Work out the finished part from the listing and answer in its coordinate system (mm). Round coordinates to 2 decimals unless told otherwise and drop trailing zeros. Write each loop counter-clockwise with the first axis right and the second up, starting at its lowest first coordinate (ties: lowest second). Pieces come first, ordered by that corner, then holes. Notation, with made-up numbers: (-35, 74) -> (-3, 74) arc R23 cw to (-3, 108) -> close; hole circle Ø4 at (-39.5, 59). An arc over 180 degrees is marked (long way). Answer as a JSON object with one key per item and string values. Group by question number.
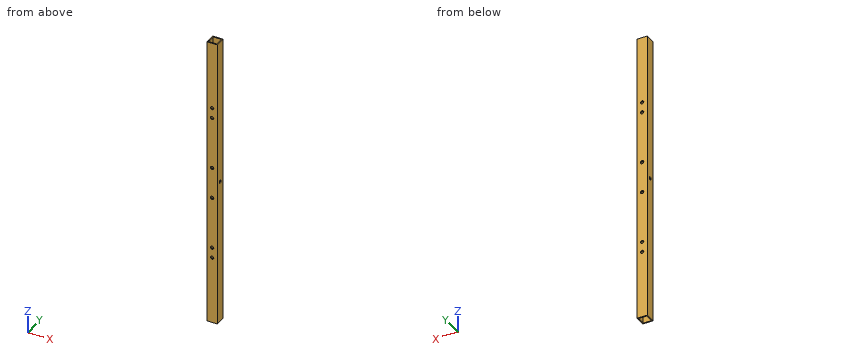
from build123d import *

# Parameters (mm, degrees)
SKETCH1_W           = 10
SKETCH1_H           = 10
SKETCH1_W_2         = 8
SKETCH1_H_2         = 8
BOSS_EXTRUDE1_DEPTH = 280
CUT_EXTRUDE1_REACH  = 282.223
SKETCH2_R           = 1.6
CUT_EXTRUDE2_REACH  = 282.223
SKETCH3_R           = 1.6


with BuildPart() as part:
    # Sketch1 → Boss-Extrude1 (new body)
    with BuildSketch(Plane.XY):
        Rectangle(SKETCH1_W, SKETCH1_H)
        Rectangle(SKETCH1_W_2, SKETCH1_H_2, mode=Mode.SUBTRACT)
    extrude(amount=BOSS_EXTRUDE1_DEPTH)

    # Cut-Extrude1: up to this face of the body (flat: up to its plane)
    cut_extrude1_end = Plane(part.part.faces().sort_by_distance((-5, 0, 140))[0])
    # Sketch2 → Cut-Extrude1 (cut, up to the picked face)
    with BuildSketch(Plane(origin=(5, 0, 0), x_dir=(0, 0, -1), z_dir=(1, 0, 0)), mode=Mode.PRIVATE) as cut_extrude1_sk1:
        with Locations(Location((-140, 0, 0), (0, 0, 90))):
            Circle(SKETCH2_R)
    cut_extrude1_tool1 = split(extrude(cut_extrude1_sk1.sketch, amount=-CUT_EXTRUDE1_REACH, mode=Mode.PRIVATE), bisect_by=cut_extrude1_end, keep=Keep.BOTH, mode=Mode.PRIVATE)
    add(cut_extrude1_tool1.solids().sort_by(Axis((5, 0, 140), (-1, 0, 0)))[0], mode=Mode.SUBTRACT)

    # Cut-Extrude2: up to this face of the body (flat: up to its plane)
    cut_extrude2_end = Plane(part.part.faces().sort_by_distance((0, -5, 140))[0])
    # Sketch3 → Cut-Extrude2 (cut, up to the picked face)
    with BuildSketch(Plane(origin=(0, 5, 0), x_dir=(1, 0, 0), z_dir=(0, 1, 0)), mode=Mode.PRIVATE) as cut_extrude2_sk1:
        with Locations(Location((0, -65, 0), (0, 0, 270))):
            Circle(SKETCH3_R)
    cut_extrude2_tool1 = split(extrude(cut_extrude2_sk1.sketch, amount=-CUT_EXTRUDE2_REACH, mode=Mode.PRIVATE), bisect_by=cut_extrude2_end, keep=Keep.BOTH, mode=Mode.PRIVATE)
    # Sketch3 → Cut-Extrude2 (cut, up to the picked face)
    with BuildSketch(Plane(origin=(0, 5, 0), x_dir=(1, 0, 0), z_dir=(0, 1, 0)), mode=Mode.PRIVATE) as cut_extrude2_sk2:
        with Locations(Location((0, -75, 0), (0, 0, 270))):
            Circle(SKETCH3_R)
    cut_extrude2_tool2 = split(extrude(cut_extrude2_sk2.sketch, amount=-CUT_EXTRUDE2_REACH, mode=Mode.PRIVATE), bisect_by=cut_extrude2_end, keep=Keep.BOTH, mode=Mode.PRIVATE)
    # Sketch3 → Cut-Extrude2 (cut, up to the picked face)
    with BuildSketch(Plane(origin=(0, 5, 0), x_dir=(1, 0, 0), z_dir=(0, 1, 0)), mode=Mode.PRIVATE) as cut_extrude2_sk3:
        with Locations(Location((0, -205, 0), (0, 0, 270))):
            Circle(SKETCH3_R)
    cut_extrude2_tool3 = split(extrude(cut_extrude2_sk3.sketch, amount=-CUT_EXTRUDE2_REACH, mode=Mode.PRIVATE), bisect_by=cut_extrude2_end, keep=Keep.BOTH, mode=Mode.PRIVATE)
    # Sketch3 → Cut-Extrude2 (cut, up to the picked face)
    with BuildSketch(Plane(origin=(0, 5, 0), x_dir=(1, 0, 0), z_dir=(0, 1, 0)), mode=Mode.PRIVATE) as cut_extrude2_sk4:
        with Locations(Location((0, -215, 0), (0, 0, 270))):
            Circle(SKETCH3_R)
    cut_extrude2_tool4 = split(extrude(cut_extrude2_sk4.sketch, amount=-CUT_EXTRUDE2_REACH, mode=Mode.PRIVATE), bisect_by=cut_extrude2_end, keep=Keep.BOTH, mode=Mode.PRIVATE)
    # Sketch3 → Cut-Extrude2 (cut, up to the picked face)
    with BuildSketch(Plane(origin=(0, 5, 0), x_dir=(1, 0, 0), z_dir=(0, 1, 0)), mode=Mode.PRIVATE) as cut_extrude2_sk5:
        with Locations(Location((0, -125, 0), (0, 0, 270))):
            Circle(SKETCH3_R)
    cut_extrude2_tool5 = split(extrude(cut_extrude2_sk5.sketch, amount=-CUT_EXTRUDE2_REACH, mode=Mode.PRIVATE), bisect_by=cut_extrude2_end, keep=Keep.BOTH, mode=Mode.PRIVATE)
    # Sketch3 → Cut-Extrude2 (cut, up to the picked face)
    with BuildSketch(Plane(origin=(0, 5, 0), x_dir=(1, 0, 0), z_dir=(0, 1, 0)), mode=Mode.PRIVATE) as cut_extrude2_sk6:
        with Locations(Location((0, -155, 0), (0, 0, 270))):
            Circle(SKETCH3_R)
    cut_extrude2_tool6 = split(extrude(cut_extrude2_sk6.sketch, amount=-CUT_EXTRUDE2_REACH, mode=Mode.PRIVATE), bisect_by=cut_extrude2_end, keep=Keep.BOTH, mode=Mode.PRIVATE)
    add(cut_extrude2_tool1.solids().sort_by(Axis((0, 5, 65), (0, -1, 0)))[0], mode=Mode.SUBTRACT)
    add(cut_extrude2_tool2.solids().sort_by(Axis((0, 5, 75), (0, -1, 0)))[0], mode=Mode.SUBTRACT)
    add(cut_extrude2_tool3.solids().sort_by(Axis((0, 5, 205), (0, -1, 0)))[0], mode=Mode.SUBTRACT)
    add(cut_extrude2_tool4.solids().sort_by(Axis((0, 5, 215), (0, -1, 0)))[0], mode=Mode.SUBTRACT)
    add(cut_extrude2_tool5.solids().sort_by(Axis((0, 5, 125), (0, -1, 0)))[0], mode=Mode.SUBTRACT)
    add(cut_extrude2_tool6.solids().sort_by(Axis((0, 5, 155), (0, -1, 0)))[0], mode=Mode.SUBTRACT)


solid = part.part
1) Straight lines are drawn through the part: L1, parallel to X at y = -2.75, z = 88.5; L2, parallel to X at y = -4.7, z = 65. For each, find the intervals that lie inside material, in ascending order.
2) This flat-tipped pin is pushed along its axis until it touches: P1, Ø1.9, axis at y = 0, z = 140, coming from the +X side. Where does it stop, or does it pass through?
3) A cutting plane is placed at A-A on y = 0. Determine the outline of the cut face in (x, z).
4) A cutting plane is placed at B-B on z = 191.5. Determine the outline of the cut face in (x, y), plus the area to 3 significant figures.
Established:
{
 "1": {"L1": "x = -5 to -4, 4 to 5", "L2": "x = -5 to -1.6, 1.6 to 5"},
 "2": {"P1": "passes through"},
 "3": {"outline": "(-5, 0) -> (-4, 0) -> (-4, 138.4) -> (-5, 138.4) -> close; (-5, 141.6) -> (-4, 141.6) -> (-4, 280) -> (-5, 280) -> close; (4, 0) -> (5, 0) -> (5, 138.4) -> (4, 138.4) -> close; (4, 141.6) -> (5, 141.6) -> (5, 280) -> (4, 280) -> close"},
 "4": {"outline": "(-5, -5) -> (5, -5) -> (5, 5) -> (-5, 5) -> close; hole (-4, -4) -> (4, -4) -> (4, 4) -> (-4, 4) -> close", "area": "36.0 mm²"}
}
